For this review, use the dimensioned drawing (mm, ordinates from the lowest corner) and the shaded views. Give positions to 0.01 mm unless a question says otherwise; leave off trailing zeros. Write each loop counter-clockwise with the first axis right and the second up, starting at its lowest first coordinate (ties: lowest second). Pieces come first, ordered by that corner, then holes.
1) For P1, Ø8, axis at x = 19.5, y = 40, coming from the -Z side; P2, Ø0.5, axis at x = 32.5, z = 1, coming from the -Y side, all flat-tipped, find the tip position at first contact; note any pin that passes through.
2) We need section C-C on z = 1.15. Give the boundary of the cut face in (x, y).
3) Wall thickness on line 1 along Y through (x, z) = (13, 0.25); line 2 along X through (y, z) = (43, 1.5); line 3 along Y through (x, z) = (31.5, 0.85): over which ranges is each line inside the solid? List them lowest first.
4) We need section A-A on x = 22. Give the boundary of the cut face in (y, z).
5) We need section B-B on y = 34.5. Give the boundary of the cut face in (x, z).
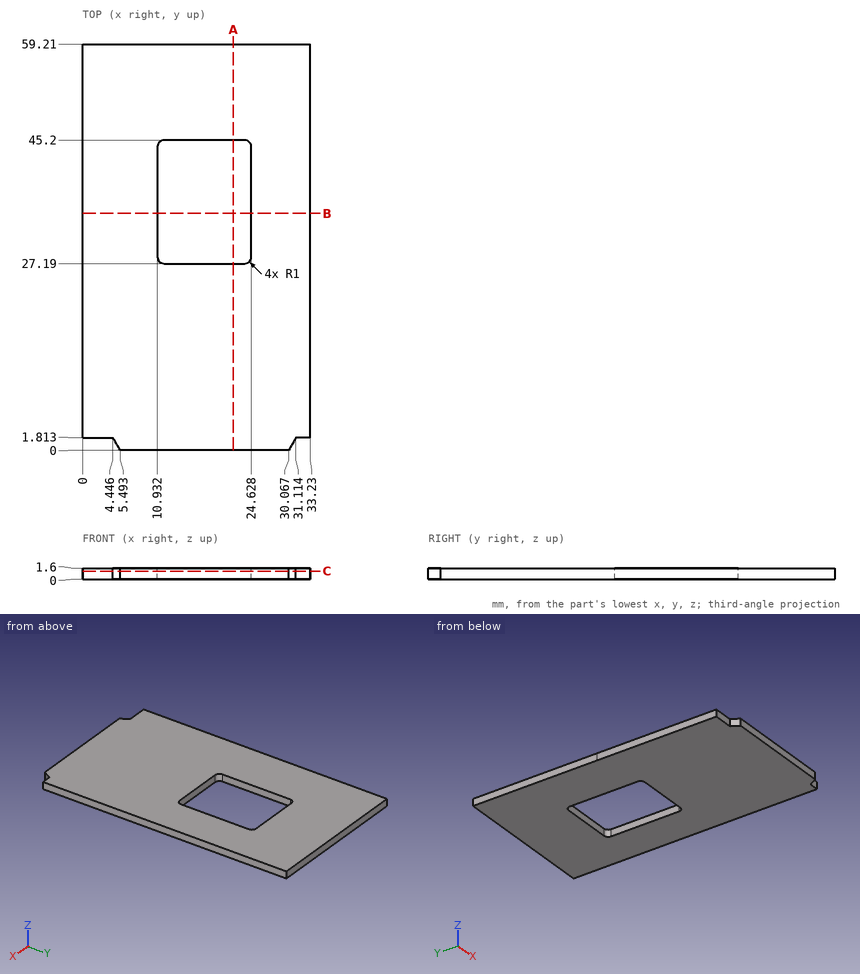
Results list:
1. P1: passes through
1. P2: stops at y = 1.81
2. outline: (0, 1.81) - (4.45, 1.81) - (5.49, 0) - (30.07, 0) - (31.11, 1.81) - (33.23, 1.81) - (33.23, 59.21) - (0, 59.21) - close; hole (10.93, 28.19) arc R1 ccw to (11.93, 27.19) - (23.63, 27.19) arc R1 ccw to (24.63, 28.19) - (24.63, 44.2) arc R1 ccw to (23.63, 45.2) - (11.93, 45.2) arc R1 ccw to (10.93, 44.2) - close
3. line 1: y = 0 to 27.19, 45.2 to 59.21
3. line 2: x = 0 to 10.93, 24.63 to 33.23
3. line 3: y = 1.81 to 59.21
4. outline: (0, 0) - (27.19, 0) - (27.19, 1.6) - (0, 1.6) - close; (45.2, 0) - (59.21, 0) - (59.21, 1.6) - (45.2, 1.6) - close
5. outline: (0, 0) - (10.93, 0) - (10.93, 1.6) - (0, 1.6) - close; (24.63, 0) - (33.23, 0) - (33.23, 1.6) - (24.63, 1.6) - close
